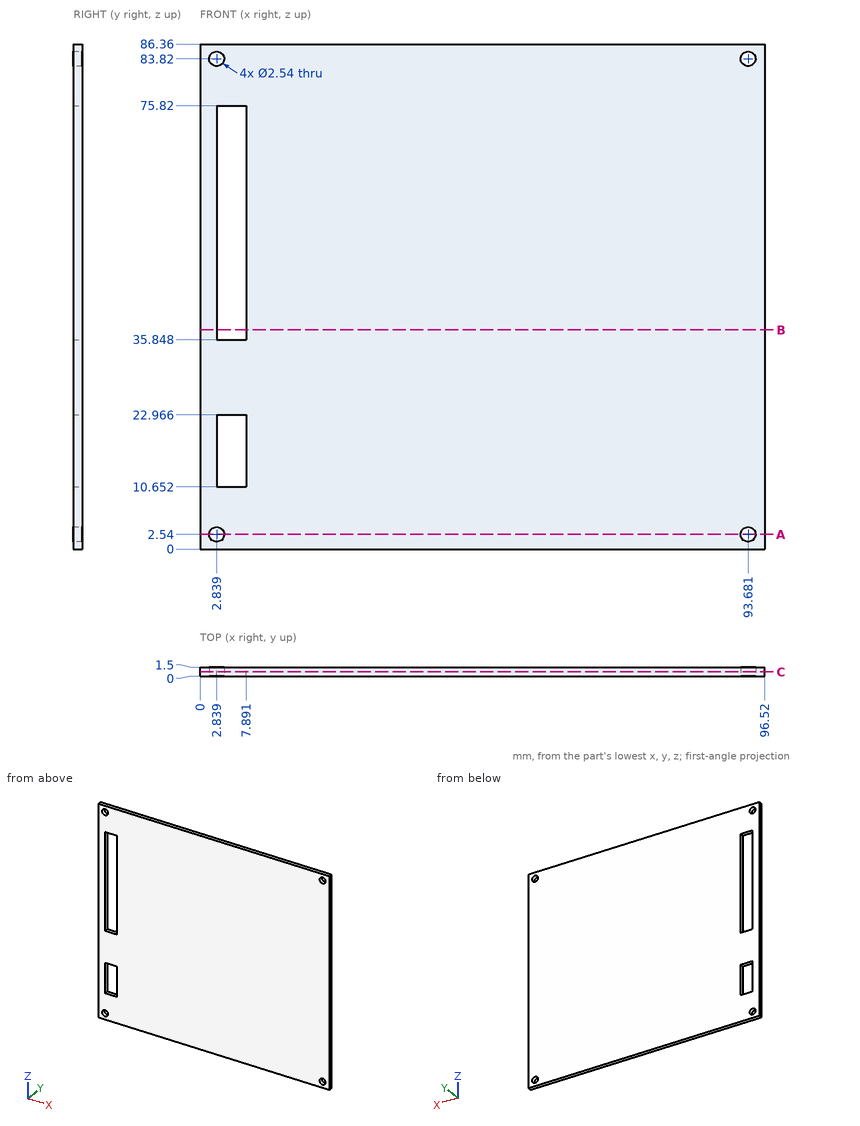
Part print with two shaded views. Sizes in mm from the minimum x, y, z corner. Give positions to 0.01 mm unless a question says otherwise; leave off trailing zeros. Order: outer loops, then holes, each group sorted by start corner. A loop starts at its lowest first (then second) coordinate and runs counter-clockwise, first axis right, second up.
(1) Saw through at B-B, the plane z = 37.5. Give the cut face in (x, y), then the cut area to 3 significant figures.
(2) Saw through at A-A, the plane z = 2.54. Give the cut face in (x, y).
(3) Saw through at C-C, the plane y = 0.7. Give the cut face in (x, z) (1 decimal).
(4) Drill centre lines: L1, parallel to X at y = 0.4, z = 2.54; L2, parallel to X at y = 1.2, z = 20; L3, parallel to Z at x = 7, y = 0.9 (1 decimal). Where is each one in solid material? Low to high.
Results found:
1. outline: (0, 0) - (2.84, 0) - (2.84, 1.5) - (0, 1.5) - close; (7.89, 0) - (96.52, 0) - (96.52, 1.5) - (7.89, 1.5) - close
1. area: 137 mm2
2. outline: (0, 0) - (1.57, 0) - (1.57, 1.5) - (0, 1.5) - close; (4.11, 0) - (92.41, 0) - (92.41, 1.5) - (4.11, 1.5) - close; (94.95, 0) - (96.52, 0) - (96.52, 1.5) - (94.95, 1.5) - close
3. outline: (0, 0) - (96.5, 0) - (96.5, 86.4) - (0, 86.4) - close; hole circle Ø2.5 at (2.8, 2.5); hole circle Ø2.5 at (2.8, 83.8); hole (2.8, 10.7) - (7.9, 10.7) - (7.9, 23) - (2.8, 23) - close; hole (2.8, 35.8) - (7.9, 35.8) - (7.9, 75.8) - (2.8, 75.8) - close; hole circle Ø2.5 at (93.7, 2.5); hole circle Ø2.5 at (93.7, 83.8)
4. L1: x = 0 to 1.57, 4.11 to 92.41, 94.95 to 96.52
4. L2: x = 0 to 2.84, 7.89 to 96.52
4. L3: z = 0 to 10.7, 23 to 35.8, 75.8 to 86.4
